Here's how the part is built. I have some questions about the finished solid (model axes, mm). Face numbers are marked on the shaded views. Give positions to 0.01 mm unless a question says otherwise; leave off trailing zeros. Write each loop counter-clockwise with the first axis right and the second up, starting at its lowest first coordinate (ties: lowest second). Pieces come first, ordered by that corner, then holes. Notation, with made-up numbers: (46, -12) - (52, -12) arc R34 cw to (52, 20) - close; hole circle Ø3 at (17, 6). An arc over 180 degrees is marked (long way). One line per item, written item: value. Start each with the question number.
1) I'm going to push a flat-ended pin straight in: P1, Ø8, axis at x = -62.5, z = 759, coming from the +Y side. Where does the tip first touch, or does it pass through?
2) Imagine slicing it at C-C on x = 153. Write out the boundary of the cut face in (y, z).
3) Imagine slicing it at A-A on x = 0. Write out the boundary of the cut face in (y, z).
4) Please list where these lines run through material, in increasing order: L1, parallel to Y at x = 0, z = 1167; L2, parallel to Z at x = 224.5, y = -426; L3, parallel to Y at x = 294, z = 143. Write a range as [from, to].
5) Imagine slicing it at D-D on y = -174. Write out the boundary of the cut face in (x, z), plus the area to 3 significant figures.
6) We'd pull the mould along X, two halves only. Please class the marked faces 1 and 2: +X half, -X half, draft (parallel to the pull), parting line (faces both ways), or undercut.
7) Imagine slicing it at B-B on y = -560.5. Write out the boundary of the cut face in (x, z), plus the area to 3 significant figures.
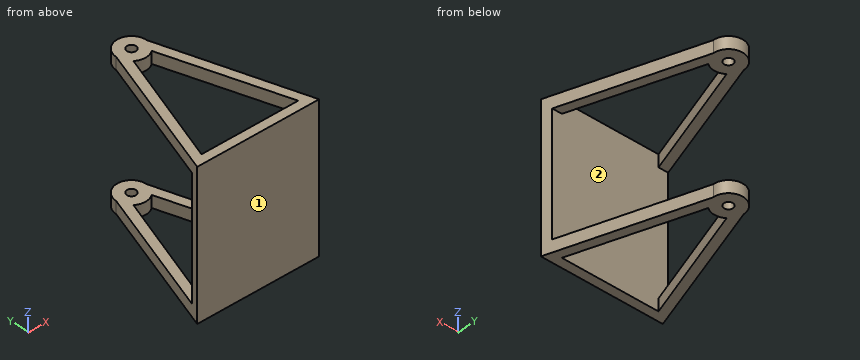
from build123d import *

# Parameters (mm, degrees)
SKETCH1_R           = 125
SKETCH1_R_2         = 37.5
BOSS_EXTRUDE1_DEPTH = 100
BOSS_EXTRUDE3_DEPTH = 500


with BuildPart() as part:
    # Sketch1 → Boss-Extrude1 (new body)
    # profile 1 of 2: a face of its own
    with BuildSketch(Plane.XY):
        with BuildLine():
            ThreePointArc((-75, -100), (-111.803398875, -55.901699437), (-125, 0))
            Line((-125, 0), (-500, -1139.901311518))
            Line((-500, -1139.901311518), (500, -1139.901311518))
            Line((500, -1139.901311518), (125, 0))
            ThreePointArc((125, 0), (111.803398875, -55.901699437), (75, -100))
            Line((75, -100), (396.372608044, -1064.901311518))
            Line((396.372608044, -1064.901311518), (-396.372608044, -1064.901311518))
            Line((-396.372608044, -1064.901311518), (-75, -100))
        make_face()
    # profile 2 of 2: a face of its own
    with BuildSketch(Plane.XY):
        Circle(SKETCH1_R)
        Circle(SKETCH1_R_2, mode=Mode.SUBTRACT)
    extrude(amount=BOSS_EXTRUDE1_DEPTH)

    # Sketch3 → Boss-Extrude3 (add)
    with BuildSketch(Plane.XY.offset(100)):
        Polygon((-500, -1139.901311518), (-475.326811439, -1064.901311518), (475.326811439, -1064.901311518), (500, -1139.901311518), align=None)
    extrude(amount=BOSS_EXTRUDE3_DEPTH)

    # Mirror2: part across plane


with BuildPart() as part_1:
    add(part.part)
    add(part.part.mirror(Plane.XY.offset(600)))


solid = part_1.part
Numbers:
1. P1: y = -1064.9
2. outline: (-1139.9, 0) - (-1064.9, 0) - (-1064.9, 1200) - (-1139.9, 1200) - close; (-334.19, 0) - (-85.11, 0) - (-85.11, 100) - (-334.19, 100) - close; (-334.19, 1100) - (-85.11, 1100) - (-85.11, 1200) - (-334.19, 1200) - close
3. outline: (-1139.9, 0) - (-1064.9, 0) - (-1064.9, 1200) - (-1139.9, 1200) - close; (-125, 0) - (-37.5, 0) - (-37.5, 100) - (-125, 100) - close; (-125, 1100) - (-37.5, 1100) - (-37.5, 1200) - (-125, 1200) - close; (37.5, 0) - (125, 0) - (125, 100) - (37.5, 100) - close; (37.5, 1100) - (125, 1100) - (125, 1200) - (37.5, 1200) - close
4. L1: [-1139.9, -1064.9], [-125, -37.5], [37.5, 125]
4. L2: [0, 100], [1100, 1200]
4. L3: [-1139.9, -1064.9]
5. outline: (-182.24, 0) - (-99.65, 0) - (-99.65, 100) - (-182.24, 100) - close; (-182.24, 1100) - (-99.65, 1100) - (-99.65, 1200) - (-182.24, 1200) - close; (99.65, 0) - (182.24, 0) - (182.24, 100) - (99.65, 100) - close; (99.65, 1100) - (182.24, 1100) - (182.24, 1200) - (99.65, 1200) - close
5. area: 33,000 mm^2
6. face 1: draft
6. face 2: undercut
7. outline: (-309.39, 0) - (-228.38, 0) - (-228.38, 100) - (-309.39, 100) - close; (-309.39, 1100) - (-228.38, 1100) - (-228.38, 1200) - (-309.39, 1200) - close; (228.38, 0) - (309.39, 0) - (309.39, 100) - (228.38, 100) - close; (228.38, 1100) - (309.39, 1100) - (309.39, 1200) - (228.38, 1200) - close
7. area: 32,400 mm^2
